Verification items for this drawing (mm, ordinates from the low corner). Coordinates: 2 decimals unless noted, no trailing zeros. Order: outer loops, then holes, each group sorted by start corner. A loop starts at its lowest first (then second) coordinate and runs counter-clockwise, first axis right, second up.
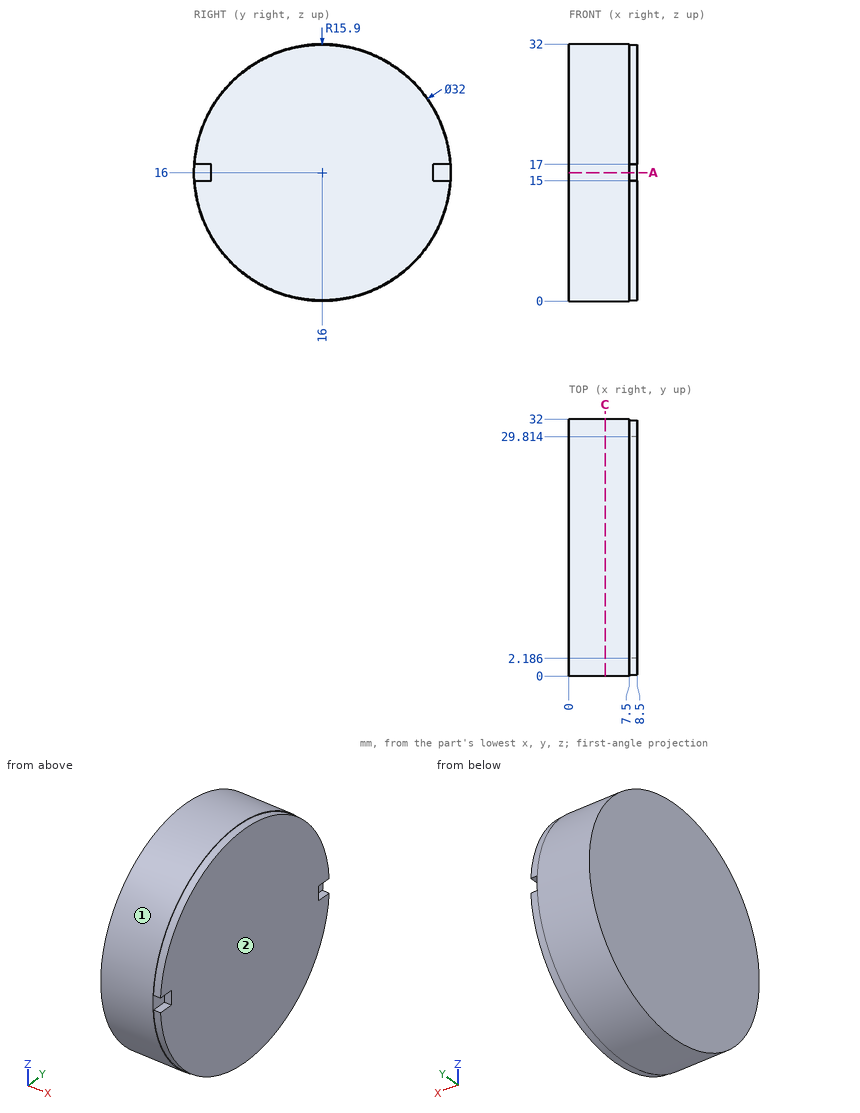
(1) Go/stop test with flat-tipped pins: P1, Ø0.5, axis at x = 8, z = 16, coming from the +Y side; P2, Ø0.8, axis at x = 8, z = 16, coming from the -Y side; P3, Ø0.8, axis at x = 8, y = 31, coming from the +Z side. Record where each tip stops, or that it passes through.
Filled in:
P1: stops at y = 29.81
P2: stops at y = 2.19
P3: stops at z = 22.3
(2) Release check for a two-part mould opening along Y. For the marked faces 1 and 2 record: +Y half, -Y half, draft (parallel to the pull), parting line (faces both ways), or undercut.
Filled in:
face 1: parting line
face 2: draft
(3) Cross-section at A-A (z = 16). Enter the section's corners in (x, y), and give its area (3 significant figures).
Filled in:
outline: (0, 0) - (7.5, 0) - (7.5, 2.19) - (8.5, 2.19) - (8.5, 29.81) - (7.5, 29.81) - (7.5, 32) - (0, 32) - close
area: 268 mm2
(4) Thickness scan on probe 1 along Y at (x, z) = (3.25, 18); probe 2 along Z at (x, y) = (1.25, 16.5); probe 3 along Y at (x, z) = (3.5, 16). Record the ranges inside material, lowest first.
Filled in:
probe 1: y = 0.13 to 31.87
probe 2: z = 0.01 to 31.99
probe 3: y = 0 to 32
(5) Cross-section at C-C (x = 4.5). Enter the section's corners in (y, z), and give its area (3 significant figures).
Filled in:
outline: circle Ø32 at (16, 16)
area: 804 mm2
